Read the model definition and answer for the solid it produces. Units are mm, in the model's axes. Coordinates: 2 decimals unless noted, no trailing zeros. Write each loop counter-clockwise with the first axis right and the second up, starting at its lowest first coordinate (ties: lowest second). Pieces come first, ordered by that corner, then holes. Notation, with made-up numbers: (75.25, -26.5) -> (79.25, -26.5) arc R24 ccw to (79.25, 11.5) -> close; hole circle Ø9 at (41, -27). An arc over 180 degrees is marked (long way). Return JSON: item names as keys, results as strings.
from build123d import *

# Parameters (mm, degrees)
SKETCH1_R           = 139.7
BOSS_EXTRUDE1_DEPTH = 3
SKETCH2_R           = 3
CUT_EXTRUDE1_DEPTH  = 4
SKETCH3_R           = 7.5
CUT_EXTRUDE2_DEPTH  = 4


with BuildPart() as part:
    # Sketch1 → Boss-Extrude1 (new body)
    with BuildSketch(Plane.XY):
        Circle(SKETCH1_R)
    extrude(amount=BOSS_EXTRUDE1_DEPTH)

    # Sketch2 → Cut-Extrude1 (cut, through all)
    with BuildSketch(Plane.XY.offset(3)):
        with Locations((0, 43.980361528)):
            Circle(SKETCH2_R)
        with Locations((31.098811876, 31.098811876)):
            Circle(SKETCH2_R)
        with Locations((43.980361528, 0)):
            Circle(SKETCH2_R)
        with Locations((31.098811876, -31.098811876)):
            Circle(SKETCH2_R)
        with Locations((0, -43.980361528)):
            Circle(SKETCH2_R)
        with Locations((-31.098811876, -31.098811876)):
            Circle(SKETCH2_R)
        with Locations((-43.980361528, 0)):
            Circle(SKETCH2_R)
        with Locations((-31.098811876, 31.098811876)):
            Circle(SKETCH2_R)
        with BuildLine():
            Line((-3, -25), (-3, 25))
            ThreePointArc((-3, 25), (0, 28), (3, 25))
            Line((3, 25), (3, -25))
            ThreePointArc((3, -25), (0, -28), (-3, -25))
        make_face()
    extrude(amount=-CUT_EXTRUDE1_DEPTH, mode=Mode.SUBTRACT)

    # Sketch3 → Cut-Extrude2 (cut, through all)
    with BuildSketch(Plane.XY.offset(3)):
        with Locations((-52, -64.5)):
            Circle(SKETCH3_R)
        with Locations((-55, -93.5)):
            Circle(SKETCH3_R)
        with Locations((52, 64.5)):
            Circle(SKETCH3_R)
        with Locations((55, 93.5)):
            Circle(SKETCH3_R)
        with Locations((52, -64.5)):
            Circle(SKETCH3_R)
        with Locations((49, -93.5)):
            Circle(SKETCH3_R)
        with Locations((-52, 64.5)):
            Circle(SKETCH3_R)
        with Locations((-49, 93.5)):
            Circle(SKETCH3_R)
    extrude(amount=-CUT_EXTRUDE2_DEPTH, mode=Mode.SUBTRACT)


solid = part.part
1. The part is cut by section A-A (y = -93.5). Determine the outline of the cut face in (x, z), then the cut area to 3 significant figures.
Taken from the geometry:
{"outline": "(-103.8, 0) -> (-62.5, 0) -> (-62.5, 3) -> (-103.8, 3) -> close; (-47.5, 0) -> (41.5, 0) -> (41.5, 3) -> (-47.5, 3) -> close; (56.5, 0) -> (103.8, 0) -> (103.8, 3) -> (56.5, 3) -> close", "area": "533 mm2"}
2. The part is cut by section D-D (y = 115). Determine the outline of the cut face in (x, z).
Taken from the geometry:
{"outline": "(-79.32, 0) -> (79.32, 0) -> (79.32, 3) -> (-79.32, 3) -> close"}
3. For a pull along Y with two mould halves and no side action, classify faces 1 (the face through (-110.86, -85.01, 1.48)), 2 (the face through (-2, -29, 0)), 3 (the face through (-41.12, 0.9, 1.52)) as +Y half, -Y half, draft (parallel to the pull), parting line (faces both ways), or undercut.
Taken from the geometry:
{"face 1": "parting line", "face 2": "draft", "face 3": "undercut"}
4. Consider L1, parallel to Y at x = 46, z = 2.45; L2, parallel to X at y = 69.5, z = 2.1; L3, parallel to Y at x = -55, z = 0.75. Determine where each line is inside the solid, lowest interval first.
Taken from the geometry:
{"L1": "y = -131.91 to -100.37, -86.63 to -69, -60 to -2.22, 2.22 to 60, 69 to 131.91", "L2": "x = -121.19 to -57.59, -46.41 to 46.41, 57.59 to 121.19", "L3": "y = -128.42 to -101, -86 to -71.37, -57.63 to 57.63, 71.37 to 89, 98 to 128.42"}
5. The part is cut by section C-C (x = 119). Determine the outline of the cut face in (y, z).
Taken from the geometry:
{"outline": "(-73.18, 0) -> (73.18, 0) -> (73.18, 3) -> (-73.18, 3) -> close"}
6. Flat-ended cylindrical pins translate along their axes: pin 1 Ø3.5 at (x, y) = (31.1, 31.1) entering from +Z; pin 2 Ø1 at (y, z) = (92, 1) entering from -X. Find the tip coordinate at first contact, or state that the pin passes through.
Taken from the geometry:
{"pin 1": "passes through", "pin 2": "stops at x = -105.56"}
7. The part is cut by section B-B (z = 1.35). Count the separate pieces of the cut face and the enclosed holes in it, then the cut area to 3 significant figures.
Taken from the geometry:
{"separate pieces": "1", "enclosed holes": "17", "area": "59,300 mm2"}
